Check sheet for the modelled part. Datum: model origin and axes. Units: mm. A direction names the side the tool comes from. Coordinates: 2 decimals unless noted, no trailing zeros. Write each loop counter-clockwise with the first axis right and the second up, starting at its lowest first coordinate (ties: lowest second). Pieces come first, ordered by that corner, then holes. Notation, with made-up numbers: (53, 48) - (88, 48) arc R38 cw to (88, 87) - close; hole circle Ø9 at (-28.75, -34). An arc over 180 degrees is marked (long way). Use one line per item in the form item = value. Start each with the question number.
1. Cross-section at D-D on x = 20. Record the boundary of the cut face in (y, z), then the cut area to 3 significant figures.
2. Draft check along Z on faces 4 (the face through (-1.5, 2.36, -0.07)), 5 (the face through (-5.149, 0.76, -23.185)), 6 (the face through (-15.94, 5.95, -10.44)). Enter one of: +Z half, -Z half, draft (parallel to the pull), parting line (faces both ways), or undercut.
3. Scan lines: line 1 along Y through (x, z) = (19, -12.5); line 2 along Z through (x, y) = (0, 4.25); line 3 along Z through (x, y) = (0, 2.2). Record each from-to range of solid material in increasing order.
4. Cross-section at C-C on y = 3. Record the boundary of the cut face in (x, z), then the cut area to 3 significant figures.
5. Go/stop test with flat-tipped pins: pin 1 Ø3 at (x, y) = (17.5, 7) entering from -Z; pin 2 Ø3 at (y, z) = (6.5, 10) entering from -X; pin 3 Ø6 at (x, y) = (5, 3) entering from +Z; pin 4 Ø2.5 at (x, z) = (0, 0) entering from +Y. Record where each tip stops, or that it passes through.
6. Tool access check on faces 1 (the face through (15.94, 4.45, -10.44)), 2 (the face through (-5, 0, 0)), 3 (the face through (-1.2, 4.65, 1.2)). Record the directions out of +Z, -Z, +X, -X, +Y, -Y that give a thin tool (end or side, any length) a straight path to the whole face; none if there is none.
```python
from build123d import *

# Parameters (mm, degrees)
SKETCH2_R          = 1.5
CUT_EXTRUDE1_DEPTH = 5.65


with BuildPart() as part:
    # Sketch1 → Revolve1 (revolve)
    with BuildSketch(Plane.XY):
        Polygon((0, 0), (23.75, 0), (23.75, 1.5), (18.9, 1.5), (18.9, 4.45), (23.75, 4.45), (23.75, 5.95), (18.9, 5.95), (18.9, 8.9), (23.75, 8.9), (23.75, 10.4), (17.4, 10.4), (17.4, 2.4), (5, 2.4), (5, 4.65), (0, 4.65), align=None)
    revolve(axis=Axis((0, 4.65, 0), (0, -1, 0)))

    # Sketch2 → Cut-Extrude1 (cut, through all)
    with BuildSketch(Plane(origin=(0, 4.65, 0), x_dir=(1, 0, 0), z_dir=(0, 1, 0))):
        Circle(SKETCH2_R)
    extrude(amount=-CUT_EXTRUDE1_DEPTH, mode=Mode.SUBTRACT)


solid = part.part
```
Final values:
q1.outline = (0, -12.81) - (1.5, -12.81) - (1.5, 12.81) - (0, 12.81) - close; (4.45, -12.81) - (5.95, -12.81) - (5.95, 12.81) - (4.45, 12.81) - close; (8.9, -12.81) - (10.4, -12.81) - (10.4, 12.81) - (8.9, 12.81) - close
q1.area = 115 mm²
q2.face_4 = undercut
q2.face_5 = parting line
q2.face_6 = draft
q3.line_1 = 0 to 1.5, 4.45 to 5.95, 8.9 to 10.4
q3.line_2 = -18.9 to -17.4, -5 to -1.5, 1.5 to 5, 17.4 to 18.9
q3.line_3 = -18.9 to -1.5, 1.5 to 18.9
q4.outline = circle Ø37.8 at (0, 0); circle Ø10 at (0, 0); hole circle Ø34.8 at (0, 0); hole circle Ø3 at (0, 0)
q4.area = 243 mm²
q5.pin_1 = -17.15
q5.pin_2 = -22.14
q5.pin_3 = 23.63
q5.pin_4 = through
q6.face_1 = none
q6.face_2 = +Z, -Z, +X, -X, -Y
q6.face_3 = +Y
